Verification items for the finished model (mm, model axes). A direction names the side the tool comes from. Coordinates: 2 decimals unless noted, no trailing zeros. Loops run counter-clockwise (first coordinate to the right, second up) from the corner with the lowest first, then second, coordinate; pieces in that order, holes last.
Q1. Access from +Z, -Z, +X, -X, +Y, -Y to the whole of each face (thin tool, end or side, straight path). Record for faces 5 (the face through (99, 115, 187)), 6 (the face through (-401, 71, 225)), 7 (the face through (0, 69, 188)), 8 (the face through (-401, 25, 187)).
Q2. Mould release check, pull along X, two halves, no side actions. Record for faces 1 (the face through (99, 71, 225)), 2 (the face through (200, 68, 86)), 3 (the face through (-155, 72, 150)), 4 (the face through (-300, 69, 188)): +X half, -X half, draft (parallel to the pull), parting line (faces both ways), or undercut.
Q3. Go/stop test with a flat-tipped pin: P1, Ø22.5, axis at x = -372.5, z = 186, coming from the -Y side. Record where the tip stops, or that it passes through.
Q4. Material ranges on probe 1 along Z at (x, y) = (-267.5, -63.5); probe 2 along Y at (x, z) = (-447.5, 208.5), recorded low to high.
Q5. Sectioned sample at D-D (x = -22.5). Enter the section's corners in (y, z).
Q6. Sectioned sample at B-B (y = 33). Enter the section's corners in (x, z).
Q7. Sectioned sample at A-A (z = 204). Enter the section's corners in (x, y).
Q8. Sectioned sample at C-C (x = 118.5). Enter the section's corners in (y, z), then the cut area to 4 significant figures.
```python
from build123d import *

# Parameters (mm, degrees)
SKETCH1_W           = 700
SKETCH1_H           = 340
BASE_EXTRUDE_DEPTH  = 150
SKETCH2_W           = 700
SKETCH2_H           = 90
BOSS_EXTRUDE1_DEPTH = 75
SKETCH3_W           = 300
SKETCH3_H           = 100
CUT_EXTRUDE1_DEPTH  = 75


with BuildPart() as part:
    # Sketch1 → Base-Extrude (new body)
    with BuildSketch(Plane.XY):
        with Locations((-150, 70)):
            Rectangle(SKETCH1_W, SKETCH1_H)
    extrude(amount=BASE_EXTRUDE_DEPTH)

    # Sketch2 → Boss-Extrude1 (add)
    with BuildSketch(Plane.XY.offset(150)):
        with Locations((-150, 70)):
            Rectangle(SKETCH2_W, SKETCH2_H)
    extrude(amount=BOSS_EXTRUDE1_DEPTH)

    # Sketch3 → Cut-Extrude1 (cut)
    with BuildSketch(Plane.XY.offset(225)):
        with Locations((-150, 70)):
            Rectangle(SKETCH3_W, SKETCH3_H)
    extrude(amount=-CUT_EXTRUDE1_DEPTH, mode=Mode.SUBTRACT)


solid = part.part
```
Geometry check:
1. face 5: +Z, +X, -X, +Y
1. face 6: +Z, +X, -X, +Y, -Y
1. face 7: +Z, +Y, -Y
1. face 8: +Z, +X, -X, -Y
2. face 1: draft
2. face 2: +X half
2. face 3: undercut
2. face 4: undercut
3. P1: stops at y = 25
4. probe 1: z = 0 to 150
4. probe 2: y = 25 to 115
5. outline: (-100, 0) - (240, 0) - (240, 150) - (-100, 150) - close
6. outline: (-500, 0) - (200, 0) - (200, 225) - (0, 225) - (0, 150) - (-300, 150) - (-300, 225) - (-500, 225) - close
7. outline: (-500, 25) - (-300, 25) - (-300, 115) - (-500, 115) - close; (0, 25) - (200, 25) - (200, 115) - (0, 115) - close
8. outline: (-100, 0) - (240, 0) - (240, 150) - (115, 150) - (115, 225) - (25, 225) - (25, 150) - (-100, 150) - close
8. area: 57,750 mm2
